Check sheet for the modelled part. Datum: model origin and axes. Units: mm. Coordinates: 2 decimals unless noted, no trailing zeros. Order: outer loops, then holes, each group sorted by start corner. A loop starts at its lowest first (then second) coordinate and runs counter-clockwise, first axis right, second up.
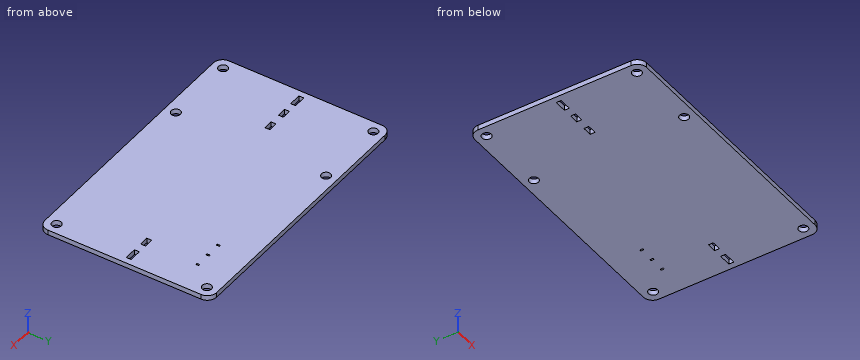
Autodesk Inventor part; units mm, degrees
ref_plane "YZ Plane" through (0, 0, 0) normal (1, 0, 0) x (0, 1, 0)
ref_plane "XZ Plane" through (0, 0, 0) normal (0, 1, 0) x (-1, 0, 0)
ref_plane "XY Plane" through (0, 0, 0) normal (0, 0, 1) x (1, 0, 0)
sketch "Sketch1" plane through (0, 0, 0) normal (0, 0, 1) x (1, 0, 0)
  line L0 (-41, -28) -> (41, -28)
  line L1 (44, -25) -> (44, 25)
  line L2 (41, 28) -> (-41, 28)
  line L3 (-44, 25) -> (-44, -25)
  line L4 (-44, -28) -> (44, 28) construction
  line L5 (44, -28) -> (-44, 28) construction
  arc A0 (-41, 28) -> (-44, 25) centre (-41, 25) ccw
  arc A1 (44, 25) -> (41, 28) centre (41, 25) ccw
  arc A2 (41, -28) -> (44, -25) centre (41, -25) ccw
  arc A3 (-44, -25) -> (-41, -28) centre (-41, -25) ccw
  point P0 (0, 0)
  dimension "d0" = 88
  dimension "d1" = 56
  dimension "d2" = 3
extrude "Extrusion1" add sketch "Sketch1" along normal blind 1.6
sketch "Sketch2" plane through (0, 0, 1.6) normal (0, 0, 1) x (1, 0, 0)
  line L0 (-42, -0.8) -> (-38, -0.8)
  line L1 (-38, -0.8) -> (-38, 0.8)
  line L2 (-38, 0.8) -> (-42, 0.8)
  line L3 (-42, 0.8) -> (-42, -0.8)
  line L4 (-42, -0.8) -> (-38, 0.8) construction
  line L5 (-38, -0.8) -> (-42, 0.8) construction
  line L6 (-35, -0.8) -> (-32, -0.8)
  line L7 (-32, -0.8) -> (-32, 0.8)
  line L8 (-32, 0.8) -> (-35, 0.8)
  line L9 (-35, 0.8) -> (-35, -0.8)
  line L10 (-35, -0.8) -> (-32, 0.8) construction
  line L11 (-32, -0.8) -> (-35, 0.8) construction
  line L12 (-28.5, -0.8) -> (-25.5, -0.8)
  line L13 (-25.5, -0.8) -> (-25.5, 0.8)
  line L14 (-25.5, 0.8) -> (-28.5, 0.8)
  line L15 (-28.5, 0.8) -> (-28.5, -0.8)
  line L16 (-28.5, -0.8) -> (-25.5, 0.8) construction
  line L17 (-25.5, -0.8) -> (-28.5, 0.8) construction
  line L18 (32, -0.8) -> (35, -0.8)
  line L19 (35, -0.8) -> (35, 0.8)
  line L20 (35, 0.8) -> (32, 0.8)
  line L21 (32, 0.8) -> (32, -0.8)
  line L22 (32, -0.8) -> (35, 0.8) construction
  line L23 (35, -0.8) -> (32, 0.8) construction
  line L24 (38, -0.8) -> (42, -0.8)
  line L25 (42, -0.8) -> (42, 0.8)
  line L26 (42, 0.8) -> (38, 0.8)
  line L27 (38, 0.8) -> (38, -0.8)
  line L28 (38, -0.8) -> (42, 0.8) construction
  line L29 (42, -0.8) -> (38, 0.8) construction
  line L30 (-44, 25) -> (-44, -25)
  line L31 (44, -25) -> (44, 25)
  point P0 (0, 0)
  point P1 (-40, 0)
  point P2 (-33.5, 0)
  point P3 (-27, 0)
  point P4 (33.5, 0)
  point P5 (40, 0)
  dimension "d5" = 2
  dimension "d6" = 4
  dimension "d7" = 3
  dimension "d8" = 3
  dimension "d9" = 3.5
  dimension "d10" = 2
  dimension "d11" = 4
  dimension "d12" = 3
  dimension "d13" = 3
  dimension "d14" = 1.6
extrude "Extrusion2" cut sketch "Sketch2" against normal blind 1.6
sketch "Sketch3" plane through (0, 0, 1.6) normal (0, 0, 1) x (1, 0, 0)
  line L0 (-40.5, 24.5) -> (-17.5, 24.5)
  line L1 (-17.5, 24.5) -> (-17.5, -24.5)
  line L2 (-17.5, -24.5) -> (-40.5, -24.5)
  line L3 (-40.5, -24.5) -> (-40.5, 24.5)
  line L4 (-17.5, 24.5) -> (40.5, 24.5)
  line L5 (40.5, 24.5) -> (40.5, -24.5)
  line L6 (40.5, -24.5) -> (-17.5, -24.5)
  line L7 (-44, 25) -> (-44, -25)
  point P0 (0, 0)
  point P1 (-40.5, 0)
  point P2 (-44, 0)
  dimension "d24" = 58
  dimension "d25" = 23
  dimension "d26" = 49
  dimension "d27" = 3.5
hole "Hole1" at (-40.5, -24.5, 1.6) at (-17.5, -24.5, 1.6) at (40.5, -24.5, 1.6) at (40.5, 24.5, 1.6) at (-17.5, 24.5, 1.6) at (-40.5, 24.5, 1.6) direction (0, 0, -1) diameter 3 end through all
sketch "Sketch4" plane through (0, 0, 1.6) normal (0, 0, 1) x (1, 0, 0)
  line L0 (23.5, 16.5) -> (24, 16.5)
  line L1 (24, 16.5) -> (24, 17.5)
  line L2 (24, 17.5) -> (23.5, 17.5)
  line L3 (23.5, 17.5) -> (23.5, 16.5)
  line L4 (33.5, 16.5) -> (34, 16.5)
  line L5 (34, 16.5) -> (34, 17.5)
  line L6 (34, 17.5) -> (33.5, 17.5)
  line L7 (33.5, 17.5) -> (33.5, 16.5)
  line L8 (28.5, 16.5) -> (29, 16.5)
  line L9 (29, 16.5) -> (29, 17.5)
  line L10 (29, 17.5) -> (28.5, 17.5)
  line L11 (28.5, 17.5) -> (28.5, 16.5)
  line L12 (41, 28) -> (-41, 28)
  line L13 (44, -25) -> (44, 25)
  point P0 (0, 0)
  point P1 (28.75, 16.5)
  point P2 (23.75, 16.5)
  point P3 (33.75, 16.5)
  point P4 (34, 17)
  dimension "d28" = 0.5
  dimension "d29" = 5
  dimension "d30" = 5
  dimension "d31" = 11.5
  dimension "d32" = 1
  dimension "d33" = 10
extrude "Extrusion3" cut sketch "Sketch4" against normal through all
properties part number "PCB_1"
(1) Cross-section at B-B (z = 0.65). Count the separate pieces of the cut face and the enclosed holes in it, and give its area (3 significant figures).
Filled in:
separate pieces: 1
enclosed holes: 14
area: 4,850 mm2
(2) Go/stop test with flat-tipped pins: P1, Ø2.5, axis at x = -17.5, y = -24.5, coming from the +Z side; P2, Ø8, axis at x = 22.5, y = 17.5, coming from the -Z side. Record where each tip stops, or that it passes through.
Filled in:
P1: passes through
P2: stops at z = 0
(3) Cross-section at A-A (x = -17.5). Enter the section's corners in (y, z), and give its area (3 significant figures).
Filled in:
outline: (-28, 0) - (-26, 0) - (-26, 1.6) - (-28, 1.6) - close; (-23, 0) - (23, 0) - (23, 1.6) - (-23, 1.6) - close; (26, 0) - (28, 0) - (28, 1.6) - (26, 1.6) - close
area: 80.0 mm2
(4) Thickness scan on probe 1 along Y at (x, z) = (-17.5, 1.25); probe 2 along X at (y, z) = (-24.5, 0.75); probe 3 along Y at (x, z) = (40.5, 0.5). Record the ranges inside material, lowest first.
Filled in:
probe 1: y = -28 to -26, -23 to 23, 26 to 28
probe 2: x = -44 to -42, -39 to -19, -16 to 39, 42 to 44
probe 3: y = -28 to -26, -23 to -0.8, 0.8 to 23, 26 to 28
